Source: CAD feature listing. Evaluate the final solid. Frame: model axes, mm. A direction names the side the tool comes from. Round coordinates to 2 decimals unless told otherwise and drop trailing zeros. Order: outer loops, then holes, each group sorted by start corner. A loop starts at its lowest first (then second) coordinate and runs counter-clockwise, first axis right, second up. Notation, with made-up numbers: M 68.5,4 L 127.5,4 A25 ccw 127.5,23 Z; hole C -10,-13 d11. An arc over 180 degrees is marked long. Answer in a Markdown table with one row per item. Add a question column.
```python
from build123d import *

# Parameters (mm, degrees)
SKETCH2_R           = 10
BOSS_EXTRUDE1_DEPTH = 3
SKETCH3_R           = 6.5
SKETCH3_R_2         = 5.6
BOSS_EXTRUDE2_DEPTH = 15
BOSS_EXTRUDE3_START = -15
SKETCH4_R           = 6.5
SKETCH4_R_2         = 2.095
BOSS_EXTRUDE3_DEPTH = 3
SKETCH5_R           = 5.6
CUT_EXTRUDE1_DEPTH  = 3
SKETCH6_R           = 1.15
CUT_EXTRUDE2_DEPTH  = 4


with BuildPart() as part:
    # Sketch2 → Boss-Extrude1 (new body)
    with BuildSketch(Plane(origin=(0, 0, 0), x_dir=(0, 0, -1), z_dir=(1, 0, 0))):
        Circle(SKETCH2_R)
    extrude(amount=BOSS_EXTRUDE1_DEPTH)

    # Sketch3 → Boss-Extrude2 (add)
    with BuildSketch(Plane(origin=(0, 0, 0), x_dir=(0, 0, -1), z_dir=(1, 0, 0))):
        Circle(SKETCH3_R)
        Circle(SKETCH3_R_2, mode=Mode.SUBTRACT)
    extrude(amount=-BOSS_EXTRUDE2_DEPTH)

    # Sketch4 → Boss-Extrude3 (add)
    with BuildSketch(Plane(origin=(0, 0, 0), x_dir=(0, 0, -1), z_dir=(1, 0, 0)).offset(BOSS_EXTRUDE3_START)):
        Circle(SKETCH4_R)
        Circle(SKETCH4_R_2, mode=Mode.SUBTRACT)
    extrude(amount=BOSS_EXTRUDE3_DEPTH)

    # Sketch5 → Cut-Extrude1 (cut)
    with BuildSketch(Plane(origin=(0, 0, 0), x_dir=(0, 0, -1), z_dir=(1, 0, 0))):
        Circle(SKETCH5_R)
    extrude(amount=CUT_EXTRUDE1_DEPTH, mode=Mode.SUBTRACT)

    # Sketch6 → Cut-Extrude2 (cut, through all)
    with BuildSketch(Plane(origin=(0, 0, 0), x_dir=(0, 0, -1), z_dir=(1, 0, 0))):
        with Locations((6.01040764, 6.01040764)):
            Circle(SKETCH6_R)
        with Locations((6.01040764, -6.01040764)):
            Circle(SKETCH6_R)
        with Locations((-6.01040764, -6.01040764)):
            Circle(SKETCH6_R)
        with Locations((-6.01040764, 6.01040764)):
            Circle(SKETCH6_R)
    extrude(amount=CUT_EXTRUDE2_DEPTH, mode=Mode.SUBTRACT)


solid = part.part
```
(1) Line query: line 1 (Y direction, x = -13.5, z = 0) (3 decimals); line 2 (Z direction, x = 0.75, y = -5.75); line 3 (Y direction, x = 1.25, z = 7). Output: solid intervals per line, ascending. Write a range as from..to.
(2) Pin query (flat end, axial travel): pin 1 (1.5 mm diameter, centred on y = -2.5, z = 3.5, fed in from +X); pin 2 (6 mm diameter, centred on x = -2, z = 7.5, fed in from +Y); pin 3 (10 mm diameter, centred on y = 0, z = 0, fed in from -X); pin 4 (4 mm diameter, centred on x = 0, y = -3, fed in from -Z). Return the tip coordinate at first contact, or that it passes through.
(3) Cut plane C-C (x = -6.75). Return loops of the section in (y, z).
(4) Access query for faces 4 (the face through (1.479, 6.356, 4.914)), 5 (the face through (-12, -2.4, 0.1)), 6 (the face through (0, -7, 0)). Directions: +Z, -Z, +X, -X, +Y, -Y. A direction counts if a zero-diameter tool reaches every point of the face in a straight line with its end or side. Return the directions, or none.
(5) Draft query along Z for faces 1 (the face through (1.48, -6.71, -5.1)), 2 (the face through (1.48, -9.76, 2.17)), 3 (the face through (3, -4.3, -4.3)). Return one class per face: +Z half, -Z half, draft (parallel to the pull), parting line (faces both ways), or undercut.
(6) Cut plane D-D (y = 2.5). Return loops of the section in (x, z), and give its area (3 significant figures).
(7) Cut plane A-A (z = 0). Return loops of the section in (x, y) (3 decimals).
Answer list:
| question | item | result |
|---|---|---|
| 1 | line 1 | -6.5..-2.095, 2.095..6.5 |
| 1 | line 2 | -8.18..-7.13, -4.89..4.89, 7.13..8.18 |
| 1 | line 3 | -7.14..-6.6, -5.42..5.42, 6.6..7.14 |
| 2 | pin 1 | x = -12 |
| 2 | pin 2 | y = 8.5 |
| 2 | pin 3 | x = -15 |
| 2 | pin 4 | z = -9.95 |
| 3 | outline | C 0,0 d13; hole C 0,0 d11.2 |
| 4 | face 4 | +X, -X |
| 4 | face 5 | +X |
| 4 | face 6 | -X |
| 5 | face 1 | undercut |
| 5 | face 2 | parting line |
| 5 | face 3 | draft |
| 6 | outline | M -15,-6 L 0,-6 L 0,-9.68 L 3,-9.68 L 3,-5.01 L -12,-5.01 L -12,5.01 L 3,5.01 L 3,9.68 L 0,9.68 L 0,6 L -15,6 Z |
| 6 | area | 87.8 mm² |
| 7 | outline | M -15,-6.5 L 0,-6.5 L 0,-10 L 3,-10 L 3,-5.6 L -12,-5.6 L -12,-2.095 L -15,-2.095 Z; M -15,2.095 L -12,2.095 L -12,5.6 L 3,5.6 L 3,10 L 0,10 L 0,6.5 L -15,6.5 Z |
